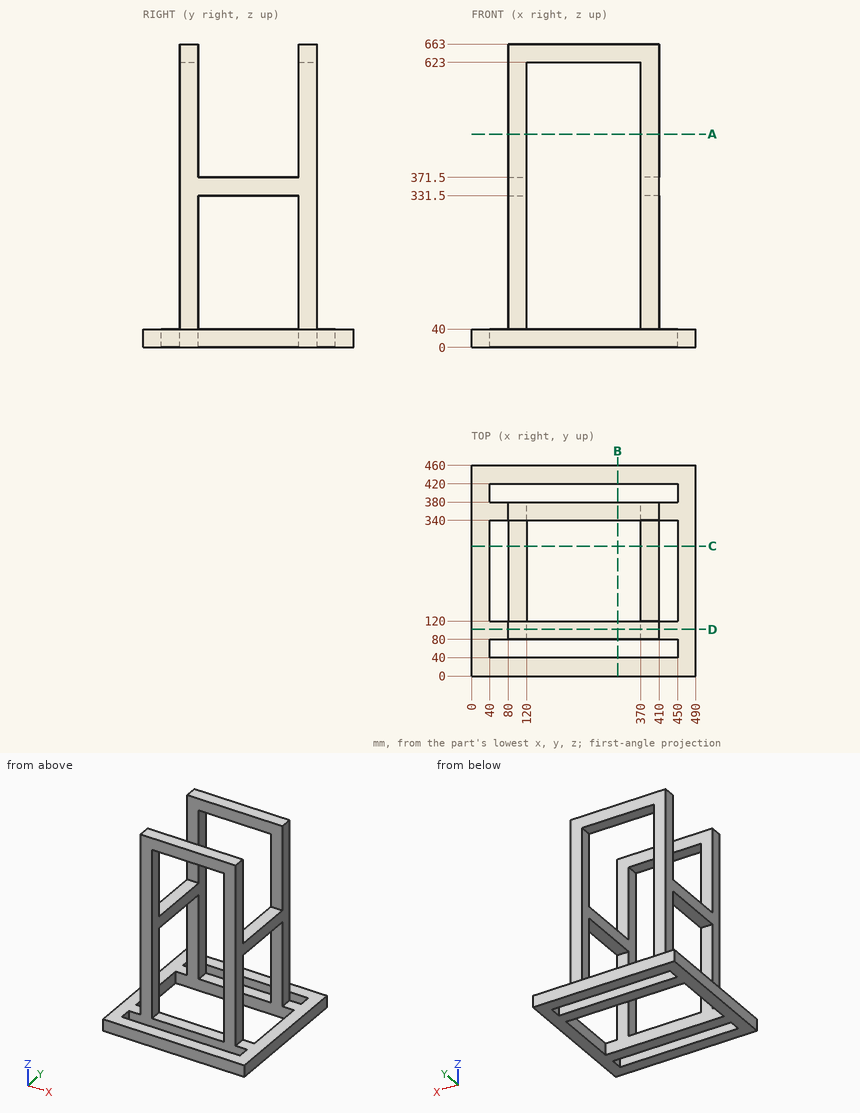
Study the drawing (mm; zero at the part's minimum x, y, z) and answer. Round coordinates to 2 decimals unless told otherwise and drop trailing zeros. Order: outer loops, then holes, each group sorted by start corner. A loop starts at its lowest first (then second) coordinate and runs counter-clockwise, first axis right, second up. Notation, with made-up numbers: (4, -4) - (53, -4) arc R22 cw to (53, 31) - close; hole circle Ø11 at (-15.75, 81.25). An arc over 180 degrees is marked (long way). Use one line per item in the form item = value. Start each with the question number.
(1) The part is cut by section A-A (z = 466). Give the vertices of the cut face in (x, y), then the cut area to 3 significant figures.
(2) The part is cut by section B-B (x = 319). Give the vertices of the cut face in (y, z), then the cut area to 3 significant figures.
(3) Flat-ended cylindrical pins translate along their axes: pin 1 Ø10 at (x, z) = (128.5, 456) entering from -Y; pin 2 Ø4 at (x, z) = (104.5, 364) entering from -Y. Find the tip coordinate at first contact, or state that the pin passes through.
(4) The part is cut by section D-D (y = 102). Give the vertices of the cut face in (x, z), then the cut area to 3 significant figures.
(5) The part is cut by section C-C (y = 283.5). Give the vertices of the cut face in (x, z), then the cut area to 3 significant figures.
(6) Find the intervals of material crossed by line 1 along Z through (x, y) = (267.5, 354.5); line 2 along Y through (x, z) = (119, 291.5); line 3 along X through (y, z) = (350, 564), in increasing order. Write a range as from..to.
Checked values:
q1.outline = (80, 80) - (120, 80) - (120, 120) - (80, 120) - close; (80, 340) - (120, 340) - (120, 380) - (80, 380) - close; (370, 80) - (410, 80) - (410, 120) - (370, 120) - close; (370, 340) - (410, 340) - (410, 380) - (370, 380) - close
q1.area = 6,400 mm^2
q2.outline = (0, 0) - (40, 0) - (40, 40) - (0, 40) - close; (80, 0) - (120, 0) - (120, 40) - (80, 40) - close; (80, 623) - (120, 623) - (120, 663) - (80, 663) - close; (340, 0) - (380, 0) - (380, 40) - (340, 40) - close; (340, 623) - (380, 623) - (380, 663) - (340, 663) - close; (420, 0) - (460, 0) - (460, 40) - (420, 40) - close
q2.area = 9,600 mm^2
q3.pin_1 = through
q3.pin_2 = 80
q4.outline = (0, 0) - (490, 0) - (490, 40) - (410, 40) - (410, 663) - (80, 663) - (80, 40) - (0, 40) - close; hole (120, 40) - (370, 40) - (370, 623) - (120, 623) - close
q4.area = 79,400 mm^2
q5.outline = (0, 0) - (40, 0) - (40, 40) - (0, 40) - close; (80, 331.5) - (120, 331.5) - (120, 371.5) - (80, 371.5) - close; (370, 331.5) - (410, 331.5) - (410, 371.5) - (370, 371.5) - close; (450, 0) - (490, 0) - (490, 40) - (450, 40) - close
q5.area = 6,400 mm^2
q6.line_1 = 0..40, 623..663
q6.line_2 = 80..120, 340..380
q6.line_3 = 80..120, 370..410
